Source: CAD feature listing. Evaluate the final solid. Frame: model axes, mm. A direction names the side the tool comes from. Give positions to 0.01 mm unless a question says otherwise; leave off trailing zeros. Write each loop counter-clockwise with the first axis right and the second up, starting at its lowest first coordinate (ties: lowest second). Pieces come first, ordered by that corner, then holes.
```python
from build123d import *

# Parameters (mm, degrees)
SKETCH1_R               = 6.35
BOSS_EXTRUDE1_DEPTH     = 5.4
HORN_START              = -2.5
HORN_DEPTH              = 2.5
SKETCH4_R               = 1.4
CUT_EXTRUDE1_DEPTH      = 21.913031822
SKETCH5_R               = 0.5
CUT_EXTRUDE2_DEPTH      = 21.913031822
LPATTERN1_COUNT         = 4
LPATTERN1_PITCH         = 3
MIRROR1_COPY_1_SKETCH_R = 0.5
MIRROR1_COPY_1_DEPTH    = 21.913031822
MIRROR1_COPY_2_SKETCH_R = 0.5
MIRROR1_COPY_2_DEPTH    = 21.913031822
MIRROR1_COPY_3_SKETCH_R = 0.5
MIRROR1_COPY_3_DEPTH    = 21.913031822


with BuildPart() as part:
    # Sketch1 → Boss-Extrude1 (new body)
    with BuildSketch(Plane(origin=(0, 0, 0), x_dir=(1, 0, 0), z_dir=(0, 1, 0))):
        with Locations(Location((0, 0, 0), (0, 0, 90))):
            Circle(SKETCH1_R)
    extrude(amount=BOSS_EXTRUDE1_DEPTH)

    # Sketch2 → horn (add)
    with BuildSketch(Plane(origin=(0, 5.4, 0), x_dir=(1, 0, 0), z_dir=(0, 1, 0)).offset(HORN_START)):
        with BuildLine():
            Line((-2.609740545, 16.990167671), (-4.891612682, 4.049027706))
            ThreePointArc((-4.891612682, 4.049027706), (0, 6.35), (4.891612682, 4.049027706))
            Line((4.891612682, 4.049027706), (2.609740545, 16.990167671))
            ThreePointArc((2.609740545, 16.990167671), (0, 19.18), (-2.609740545, 16.990167671))
        make_face()
    horn = extrude(amount=HORN_DEPTH)

    # Sketch4 → Cut-Extrude1 (cut, through all)
    with BuildSketch(Plane(origin=(0, 5.4, 0), x_dir=(-1, 0, 0), z_dir=(0, -1, 0))):
        with Locations(Location((0, 0, 0), (0, 0, 270))):
            Circle(SKETCH4_R)
    extrude(amount=CUT_EXTRUDE1_DEPTH, mode=Mode.SUBTRACT)

    # Sketch5 → Cut-Extrude2 (cut, through all)
    with BuildSketch(Plane(origin=(0, 0, 0), x_dir=(-1, 0, 0), z_dir=(0, -1, 0))):
        with Locations(Location((0, 16.53, 0), (0, 0, 90))):
            Circle(SKETCH5_R)
    cut_extrude2 = extrude(amount=-CUT_EXTRUDE2_DEPTH, mode=Mode.SUBTRACT)

    # LPattern1: Cut-Extrude2 ×4
    with Locations(*[(0, 0, i * LPATTERN1_PITCH) for i in range(1, LPATTERN1_COUNT)]):
        add(cut_extrude2, mode=Mode.SUBTRACT)

    # Mirror1: horn, Cut-Extrude2 across plane
    add(horn.mirror(Plane.XY))
    add(cut_extrude2.mirror(Plane.XY), mode=Mode.SUBTRACT)

    # Mirror1 copy 1 sketch → Mirror1 copy 1 (cut, through all)
    with BuildSketch(Plane(origin=(0, 0, -3), x_dir=(-1, 0, 0), z_dir=(0, -1, 0))):
        with Locations((0, -16.53)):
            Circle(MIRROR1_COPY_1_SKETCH_R)
    extrude(amount=-MIRROR1_COPY_1_DEPTH, mode=Mode.SUBTRACT)

    # Mirror1 copy 2 sketch → Mirror1 copy 2 (cut, through all)
    with BuildSketch(Plane(origin=(0, 0, -6), x_dir=(-1, 0, 0), z_dir=(0, -1, 0))):
        with Locations((0, -16.53)):
            Circle(MIRROR1_COPY_2_SKETCH_R)
    extrude(amount=-MIRROR1_COPY_2_DEPTH, mode=Mode.SUBTRACT)

    # Mirror1 copy 3 sketch → Mirror1 copy 3 (cut, through all)
    with BuildSketch(Plane(origin=(0, 0, -9), x_dir=(-1, 0, 0), z_dir=(0, -1, 0))):
        with Locations((0, -16.53)):
            Circle(MIRROR1_COPY_3_SKETCH_R)
    extrude(amount=-MIRROR1_COPY_3_DEPTH, mode=Mode.SUBTRACT)


solid = part.part
```
1. Section query D-D (z = 10.53). Return loops of the section in (x, y).
2. Pin query (flat end, axial travel): P1, Ø2, axis at x = -3.5, y = 1, coming from the +Z side; P2, Ø3, axis at x = 2.5, z = -9, coming from the -Y side; P3, Ø2, axis at y = 1.5, z = 1.5, coming from the +X side. Return the tip coordinate at first contact, or that it passes through.
3. Access query for faces 1 (the flat face through (3.767, 4.132, -10.429)), 2 (the cylindrical face through (-1.907, 2.062, -6.057)). Directions: +Z, -Z, +X, -X, +Y, -Y. A direction counts if a zero-diameter tool reaches every point of the face in a straight line with its end or side. Return the directions, or none.
4. Section query B-B (y = 3.6). Give the number of separate pieces and of enclosed holes in the cut face, plus the area to 3 significant figures.
5. Line query: probe 1 along Y at (x, z) = (-2.5, -15); probe 2 along X at (y, z) = (3.8, -7.53); probe 3 along X at (y, z) = (3.5, -10.53). Output: solid intervals per line, ascending.
6. Section query C-C (x = -3). Return loops of the section in (y, z), plus the area to 3 significant figures.
7. Section query A-A (z = 0). Return loops of the section in (x, y).
The answers:
1. outline: (-3.75, 2.9) - (-0.5, 2.9) - (-0.5, 5.4) - (-3.75, 5.4) - close; (0.5, 2.9) - (3.75, 2.9) - (3.75, 5.4) - (0.5, 5.4) - close
2. P1: stops at z = 5.84
2. P2: stops at y = 2.9
2. P3: stops at x = 6.33
3. face 1: -Z, +X, +Y, -Y
3. face 2: -Y
4. separate pieces: 1
4. enclosed holes: 9
4. area: 294 mm2
5. probe 1: y = 2.9 to 5.4
5. probe 2: x = -4.28 to -0.5, 0.5 to 4.28
5. probe 3: x = -3.75 to -0.5, 0.5 to 3.75
6. outline: (0, -5.6) - (2.9, -5.6) - (2.9, -14.78) - (5.4, -14.78) - (5.4, 14.78) - (2.9, 14.78) - (2.9, 5.6) - (0, 5.6) - close
6. area: 106 mm2
7. outline: (-6.35, 0) - (-1.4, 0) - (-1.4, 5.4) - (-6.35, 5.4) - close; (1.4, 0) - (6.35, 0) - (6.35, 5.4) - (1.4, 5.4) - close
